Geometry check sheet. Reference: the model listing, model coordinates, mm. Coordinates: 2 decimals unless noted, no trailing zeros. Order: outer loops, then holes, each group sorted by start corner. A loop starts at its lowest first (then second) coordinate and runs counter-clockwise, first axis right, second up. Notation, with made-up numbers: M 18.25,-33 L 28.25,-33 A9 cw 28.25,-18 Z; hole C 60,27 d7. An arc over 180 degrees is marked long. One line per item, written item: value. Start each with the question number.
1) Go/stop test with flat-tipped pins: P1, Ø3, axis at y = -2, z = -39, coming from the -X side; P2, Ø1.9, axis at x = -28, y = -2.5, coming from the -Z side (3 decimals); P3, Ø3, axis at y = -3, z = 45.5, coming from the -X side; P4, Ø2, axis at x = 16, z = 29, coming from the +Y side. Record where each tip stops, or that it passes through.
2) Thickness scan on L1, parallel to X at y = -5, z = -36.5; L2, parallel to Z at x = 41.5, y = -5.5 (3 decimals); L3, parallel to X at y = -0.5, z = -8. Record the ranges inside material, lowest first. Write a range as from..to.
3) Sectioned sample at B-B, the plane x = -3.5. Enter the section's corners in (y, z) (3 decimals), then the cut area to 3 significant figures.
4) Sectioned sample at A-A, the plane z = -17.5. Enter the section's corners in (x, y), then the cut area to 3 significant figures.
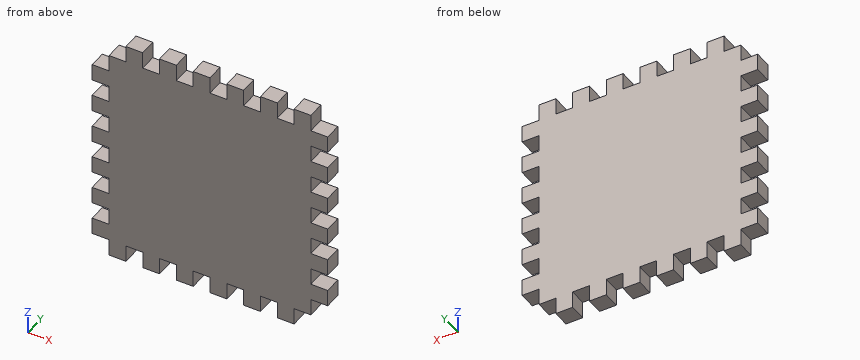
```python
from build123d import *

# Parameters (mm, degrees)
F1_DEPTH = 6.35


with BuildPart() as f1:
    # F0 (on Front) → F1 (new body)
    with BuildSketch(Plane.XZ):
        Polygon((-25.4, 47.625), (-31.75, 47.625), (-31.75, 41.275), (-38.1, 41.275), (-38.1, 34.925), (-44.47566, 34.925), (-44.47566, 28.575), (-38.109287, 28.575), (-38.109287, 22.225), (-44.47566, 22.225), (-44.47566, 15.875), (-38.109287, 15.875), (-38.109287, 9.525), (-44.47566, 9.525), (-44.47566, 3.175), (-38.109287, 3.175), (-38.1, -3.175), (-44.47566, -3.175), (-44.47566, -9.525), (-38.1, -9.525), (-38.1, -15.875), (-44.47566, -15.875), (-44.47566, -22.225), (-38.1, -22.225), (-38.07434, -28.575), (-44.47566, -28.575), (-44.47566, -34.925), (-38.07434, -34.925), (-38.07434, -41.275), (-31.72434, -41.275), (-31.72434, -34.925), (-25.37434, -34.925), (-25.37434, -41.275), (-25.32191, -41.275), (-19.02434, -41.275), (-19.02434, -34.925), (-12.67434, -34.925), (-12.67434, -41.275), (-12.450798, -41.275), (-6.32434, -41.275), (-6.32434, -34.925), (0.02566, -34.925), (0.02566, -41.275), (6.37566, -41.275), (6.37566, -34.925), (12.72566, -34.925), (12.72566, -41.275), (19.07566, -41.275), (19.07566, -34.925), (25.42566, -34.925), (25.42566, -41.275), (31.77566, -41.275), (31.77566, -34.925), (38.1, -34.925), (38.1, -28.575), (44.47566, -28.575), (44.47566, -22.225), (38.1, -22.225), (38.1, -15.875), (44.47566, -15.875), (44.47566, -9.525), (38.1, -9.525), (38.1, -3.175), (44.47566, -3.175), (44.47566, 3.175), (38.1, 3.175), (38.1, 9.525), (44.47566, 9.525), (44.47566, 15.875), (38.1, 15.875), (38.1, 22.225), (44.47566, 22.225), (44.47566, 28.575), (38.1, 28.575), (38.1, 34.925), (44.47566, 34.925), (44.47566, 41.275), (38.1, 41.275), (38.1, 47.625), (31.77566, 47.625), (31.77566, 41.275), (25.42566, 41.275), (25.42566, 47.625), (19.07566, 47.625), (19.07566, 41.275), (12.7, 41.275), (12.7, 47.625), (6.35, 47.625), (6.35, 41.275), (0, 41.275), (0, 47.625), (-6.35, 47.625), (-6.35, 41.275), (-12.7, 41.275), (-12.7, 47.625), (-19.05, 47.625), (-19.05, 41.275), (-25.4, 41.275), align=None)
    extrude(amount=F1_DEPTH)


solid = f1.part
```
Final values:
1. P1: stops at x = -38.07
1. P2: stops at z = -34.925
1. P3: stops at x = -31.75
1. P4: stops at y = 0
2. L1: x = -38.07..-31.72, -25.37..-19.02, -12.67..-6.32, 0.03..6.38, 12.73..19.08, 25.43..31.78
2. L2: z = -28.575..-22.225, -15.875..-9.525, -3.175..3.175, 9.525..15.875, 22.225..28.575, 34.925..41.275
2. L3: x = -44.48..38.1
3. outline: M -6.35,-34.925 L 0,-34.925 L 0,47.625 L -6.35,47.625 Z
3. area: 524 mm^2
4. outline: M -44.48,-6.35 L 38.1,-6.35 L 38.1,0 L -44.48,0 Z
4. area: 524 mm^2
